Geometry check sheet. Reference: the model listing, model coordinates, mm. Face numbers are marked on the shaded views. A direction names the side the tool comes from. Give positions to 0.01 mm unless a question says otherwise; leave off trailing zeros. Order: outer loops, then holes, each group sorted by start corner. A loop starts at its lowest first (then second) coordinate and runs counter-clockwise, first axis right, second up.
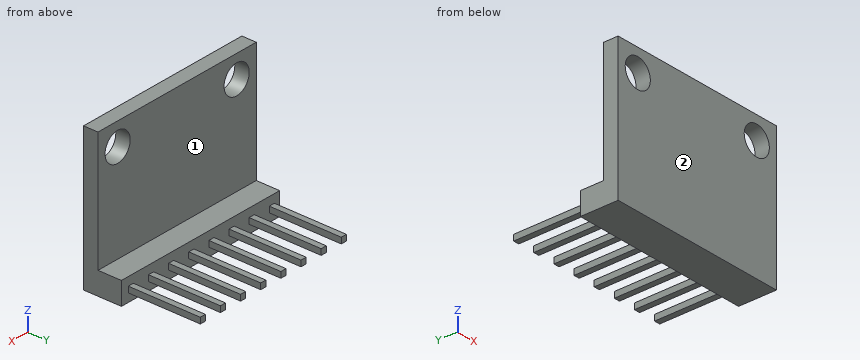
from build123d import *

# Parameters (mm, degrees)
SKETCH1_W           = 20.15
SKETCH1_H           = 15.82
BOSS_EXTRUDE1_DEPTH = 1.6
SKETCH2_R           = 1.6
CUT_EXTRUDE1_DEPTH  = 13.908668599
BOSS_EXTRUDE2_START = -1.6
SKETCH3_W           = 20.15
SKETCH3_H           = 2.5
BOSS_EXTRUDE2_DEPTH = 4.2
SKETCH5_W           = 0.65
SKETCH5_H           = 0.65
BOSS_EXTRUDE3_DEPTH = 8
LPATTERN1_COUNT     = 8
LPATTERN1_PITCH     = 2.564285714


with BuildPart() as part:
    # Sketch1 → Boss-Extrude1 (new body)
    with BuildSketch(Plane(origin=(0, 0, 0), x_dir=(1, 0, 0), z_dir=(0, 1, 0))):
        Rectangle(SKETCH1_W, SKETCH1_H)
    extrude(amount=BOSS_EXTRUDE1_DEPTH)

    # Sketch2 → Cut-Extrude1 (cut, through all)
    with BuildSketch(Plane(origin=(0, 1.6, 0), x_dir=(1, 0, 0), z_dir=(0, 1, 0))):
        with Locations(Location((-7.575, -5.41, 0), (0, 0, 270))):
            Circle(SKETCH2_R)
        with Locations(Location((7.575, -5.41, 0), (0, 0, 270))):
            Circle(SKETCH2_R)
    extrude(amount=-CUT_EXTRUDE1_DEPTH, mode=Mode.SUBTRACT)

    # Sketch3 → Boss-Extrude2 (add)
    with BuildSketch(Plane(origin=(0, 1.6, 0), x_dir=(1, 0, 0), z_dir=(0, 1, 0)).offset(BOSS_EXTRUDE2_START)):
        with Locations((0, 6.66)):
            Rectangle(SKETCH3_W, SKETCH3_H)
    extrude(amount=BOSS_EXTRUDE2_DEPTH)

    # Sketch5 → Boss-Extrude3 (add)
    with BuildSketch(Plane(origin=(0, 4.2, 0), x_dir=(1, 0, 0), z_dir=(0, 1, 0))):
        with Locations((-9.075, 6.66)):
            Rectangle(SKETCH5_W, SKETCH5_H)
    boss_extrude3 = extrude(amount=BOSS_EXTRUDE3_DEPTH)

    # LPattern1: Boss-Extrude3 ×8
    with Locations(*[(i * LPATTERN1_PITCH, 0, 0) for i in range(1, LPATTERN1_COUNT)]):
        add(boss_extrude3)


solid = part.part
Item 1: Scan lines: L1, parallel to X at y = 1.1, z = 5.41 (3 decimals); L2, parallel to Z at x = 1.25, y = 10.75 (3 decimals); L3, parallel to Y at x = 1, z = 1.5. Record each from-to range of solid material in increasing order.
Reported:
L1: x = -10.075 to -9.175, -5.975 to 5.975, 9.175 to 10.075
L2: z = -6.985 to -6.335
L3: y = 0 to 1.6
Item 2: Sectioned sample at D-D (x = 3). Enter the section's corners in (y, z), and give its area (3 significant figures).
Reported:
outline: (0, -7.91) - (4.2, -7.91) - (4.2, -5.41) - (1.6, -5.41) - (1.6, 7.91) - (0, 7.91) - close
area: 31.8 mm2
Item 3: Sectioned sample at B-B (y = 9.75). Give the number of separate pieces and of enclosed holes in the cut face, and give its area (3 significant figures).
Reported:
separate pieces: 8
enclosed holes: 0
area: 3.38 mm2
Item 4: Gauge pin test, flat ends, axial feed: pin 1 (0.7 mm diameter, centred on y = 8, z = -6.5, fed in from -X); pin 2 (0.5 mm diameter, centred on x = 3.5, y = 9, fed in from +Z) (3 decimals); pin 3 (0.7 mm diameter, centred on x = -4, y = 10, fed in from -Z) (3 decimals). Record the tip position at first contact, or that the pin passes through.
Reported:
pin 1: stops at x = -9.4
pin 2: stops at z = -6.335
pin 3: stops at z = -6.985
Item 5: Set-up check for the marked faces 1 and 2: record each of +Z, -Z, +X, -X, +Y, -Y from which the full face is reachable in a straight line by a thin tool's end or side.
Reported:
face 1: +Z, +X, -X, +Y
face 2: +Z, -Z, +X, -X, -Y
Item 6: Sectioned sample at C-C (x = 7). Enter the section's corners in (y, z).
Reported:
outline: (0, -7.91) - (4.2, -7.91) - (4.2, -5.41) - (1.6, -5.41) - (1.6, 3.92) - (0, 3.92) - close; (0, 6.9) - (1.6, 6.9) - (1.6, 7.91) - (0, 7.91) - close
Item 7: Sectioned sample at A-A (z = 5.41). Enter the section's corners in (x, y) (3 decimals), and give its area (3 significant figures).
Reported:
outline: (-10.075, 0) - (-9.175, 0) - (-9.175, 1.6) - (-10.075, 1.6) - close; (-5.975, 0) - (5.975, 0) - (5.975, 1.6) - (-5.975, 1.6) - close; (9.175, 0) - (10.075, 0) - (10.075, 1.6) - (9.175, 1.6) - close
area: 22.0 mm2
